Answer from the drawing. Dimensions are ordinates in mm from the lowest x, y and z of the part. A direction names the side the tool comes from. Give positions to 0.01 mm unless a question says otherwise; leave off trailing zeros. Order: outer loops, then holes, each group sorted by start corner. A loop starts at its lowest first (then second) coordinate and runs counter-clockwise, first axis right, second up.
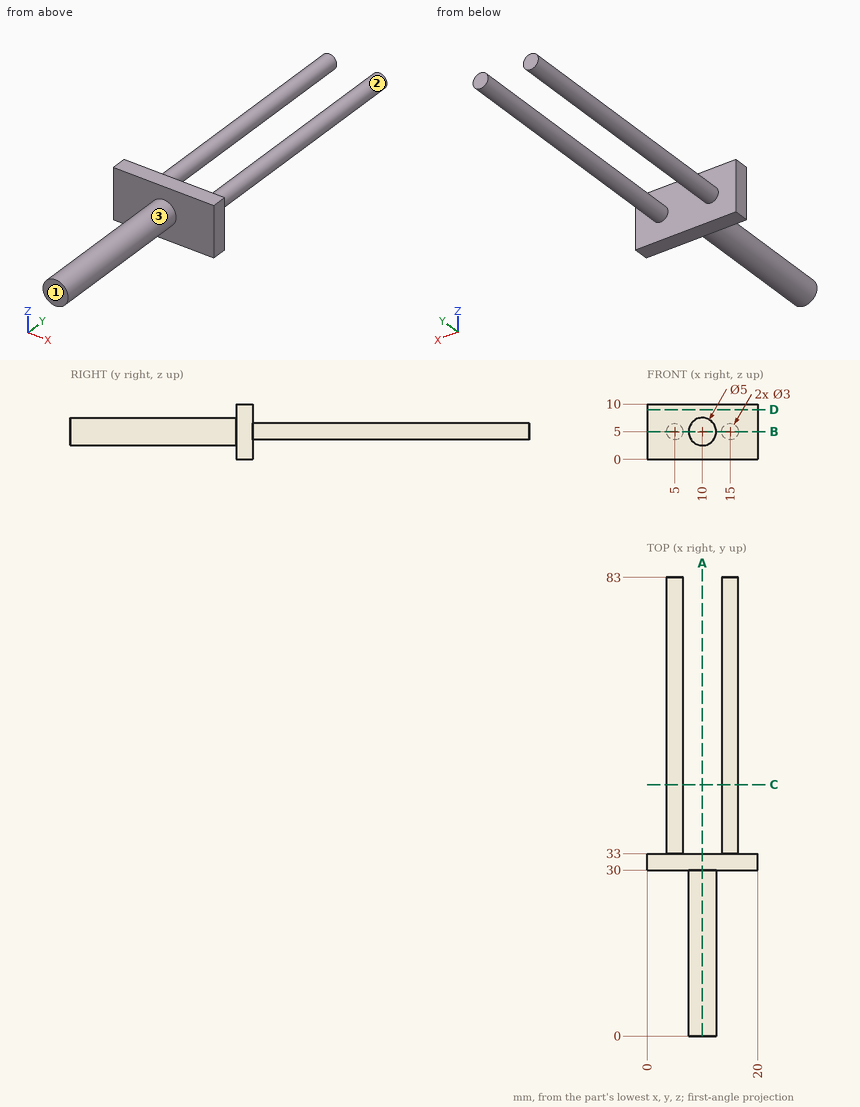
1. Which of the six approach directions +Z, -Z, +X, -X, +Y, -Y give full straight-line access (tool end or side, diameter ignored) to the marked faces 1, 2 and 3?
Findings below:
face 1: +Z, -Z, +X, -X, -Y
face 2: +Y
face 3: -Y
2. The part is cut by section C-C (y = 45.5). Write down the section's boundary in (x, z), then the cut area to 3 significant figures.
Findings below:
outline: circle Ø3 at (5, 5); circle Ø3 at (15, 5)
area: 14.1 mm2
3. The part is cut by section D-D (z = 9). Write down the section's boundary in (x, y).
Findings below:
outline: (0, 30) - (20, 30) - (20, 33) - (0, 33) - close
4. The part is cut by section B-B (z = 5). Write down the section's boundary in (x, y).
Findings below:
outline: (0, 30) - (7.5, 30) - (7.5, 0) - (12.5, 0) - (12.5, 30) - (20, 30) - (20, 33) - (16.5, 33) - (16.5, 83) - (13.5, 83) - (13.5, 33) - (6.5, 33) - (6.5, 83) - (3.5, 83) - (3.5, 33) - (0, 33) - close
5. Given P1, Ø1, axis at x = 5.5, y = 45, coming from the +Z side; P2, Ø4, axis at y = 73.5, z = 6, coming from the -X side; P3, Ø1.5, axis at y = 41.5, z = 4.5, coming from the +X side, each flat-ended and moving along its own axis, determine where each tip first touches the part or whether it passes through.
Findings below:
P1: stops at z = 6.5
P2: stops at x = 3.5
P3: stops at x = 16.5
6. The part is cut by section A-A (x = 10). Write down the section's boundary in (y, z).
Findings below:
outline: (0, 2.5) - (30, 2.5) - (30, 0) - (33, 0) - (33, 10) - (30, 10) - (30, 7.5) - (0, 7.5) - close
7. Straight lines are drawn through the part: probe 1 along Z at (x, y) = (15, 46.5); probe 2 along Y at (x, z) = (8.5, 1); probe 3 along X at (y, z) = (23.5, 4.75). For each, find the intervals that lie inside material, in ascending order.
Findings below:
probe 1: z = 3.5 to 6.5
probe 2: y = 30 to 33
probe 3: x = 7.51 to 12.49
